Build history of the part. All positions in model axes, mm. Face numbers are marked on the shaded views. A direction names the side the tool comes from. Round coordinates to 2 decimals unless told otherwise and drop trailing zeros. Write each loop counter-clockwise with the first axis right and the second up, starting at its lowest first coordinate (ties: lowest second). Pieces come first, ordered by that corner, then holes. Notation, with made-up numbers: (-16.5, -31) - (-9.5, -31) arc R28 ccw to (-9.5, -6) - close; hole circle Ø3 at (60.5, 82). An arc over 180 degrees is marked (long way). One line per question, with ' | ' between items.
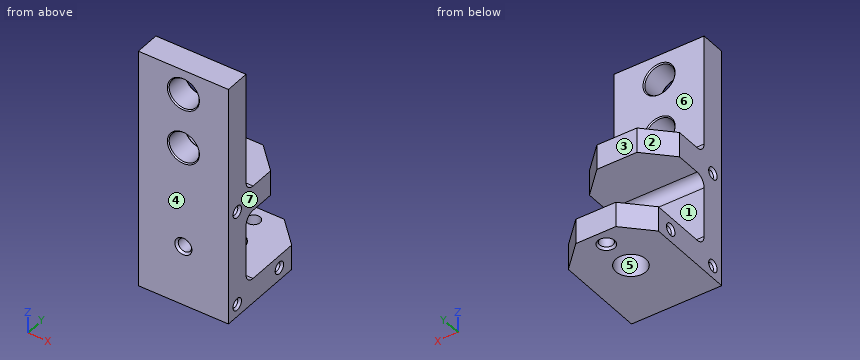
from build123d import *

# Parameters (mm, degrees)
EXTRUDE4_DEPTH                    = 57.15
EXTRUDE7_DEPTH                    = 57.15
CUT_EXTRUDE2_REACH                = 155.035
SKETCH10_R                        = 9.525
F_3_8_24_TAPPED_HOLE1_D           = 8.4328
F_3_8_24_TAPPED_HOLE1_DEPTH       = 15.875
F_3_8_24_TAPPED_HOLE1_CSINK_D     = 10.795
F_3_8_24_TAPPED_HOLE1_CSINK_ANGLE = 82
F_3_8_24_TAPPED_HOLE2_D           = 8.4328
F_3_8_24_TAPPED_HOLE2_DEPTH       = 15.875
F_3_8_24_TAPPED_HOLE2_CSINK_D     = 10.795
F_3_8_24_TAPPED_HOLE2_CSINK_ANGLE = 82
F_1_4_20_TAPPED_HOLE1_D           = 5.1054
F_1_4_20_TAPPED_HOLE1_DEPTH       = 16.51
F_1_4_20_TAPPED_HOLE1_CSINK_D     = 7.62
F_1_4_20_TAPPED_HOLE1_CSINK_ANGLE = 82
F_1_4_20_TAPPED_HOLE1_TIP         = 1.533816902
F_1_4_20_TAPPED_HOLE2_D           = 5.1054
F_1_4_20_TAPPED_HOLE2_DEPTH       = 16.51
F_1_4_20_TAPPED_HOLE2_CSINK_D     = 7.62
F_1_4_20_TAPPED_HOLE2_CSINK_ANGLE = 82
F_1_4_20_TAPPED_HOLE2_TIP         = 1.533816902
CUT_EXTRUDE3_REACH                = 155.035
F_1_2_CLEARANCE_HOLE1_AT_2_COUNT  = 2
F_1_2_CLEARANCE_HOLE1_AT_2_PITCH  = 34.925
CUT_EXTRUDE4_REACH                = 78.2
FILLET4_R                         = 6.35


with BuildPart() as part:
    # Sketch5 → Extrude4 (new body)
    with BuildSketch(Plane(origin=(0, 0, 0), x_dir=(0, 0, -1), z_dir=(1, 0, 0))):
        Polygon((0, 46.0375), (0, -7.9375), (-92.71, -7.9375), (-92.71, 7.9375), (-15.875, 7.9375), (-15.875, 46.0375), align=None)
    extrude(amount=EXTRUDE4_DEPTH)

    # Sketch9 → Extrude7 (add)
    with BuildSketch(Plane(origin=(57.15, 0, 0), x_dir=(0, 0, -1), z_dir=(1, 0, 0))):
        Polygon((0, 7.9375), (44.45, 7.9375), (44.45, 65.0875), (60.325, 65.0875), (60.325, -7.9375), (0, -7.9375), align=None)
    extrude(amount=-EXTRUDE7_DEPTH)

    # Sketch10 → Cut-Extrude2 (cut, up to next)
    with BuildSketch(Plane(origin=(0, 0, -60.325), x_dir=(-1, 0, 0), z_dir=(0, 0, -1)), mode=Mode.PRIVATE) as cut_extrude2_sk1:
        with Locations((-28.575, 33.3375)):
            Circle(SKETCH10_R)
    cut_extrude2_tool1 = extrude(cut_extrude2_sk1.sketch, amount=-CUT_EXTRUDE2_REACH, mode=Mode.PRIVATE) & part.part
    add(cut_extrude2_tool1.solids().sort_by_distance((28.575, 33.3375, -60.325))[0], mode=Mode.SUBTRACT)

    # 3/8-24 Tapped Hole1
    with Locations(Plane(origin=(0, 0, -60.325), x_dir=(-1, 0, 0), z_dir=(0, 0, -1))):
        with Locations((-28.575, 55.5625)):
            CounterSinkHole(F_3_8_24_TAPPED_HOLE1_D / 2, F_3_8_24_TAPPED_HOLE1_CSINK_D / 2, depth=F_3_8_24_TAPPED_HOLE1_DEPTH, counter_sink_angle=F_3_8_24_TAPPED_HOLE1_CSINK_ANGLE)

    # 3/8-24 Tapped Hole2
    with Locations(Plane.XZ.offset(7.9375)):
        with Locations((28.575, -22.225)):
            CounterSinkHole(F_3_8_24_TAPPED_HOLE2_D / 2, F_3_8_24_TAPPED_HOLE2_CSINK_D / 2, depth=F_3_8_24_TAPPED_HOLE2_DEPTH, counter_sink_angle=F_3_8_24_TAPPED_HOLE2_CSINK_ANGLE)

    # 1/4-20 Tapped Hole1
    with Locations(Plane.ZY):
        with Locations((-52.3875, 0), (7.9375, 0), (-52.3875, 38.1)):
            CounterSinkHole(F_1_4_20_TAPPED_HOLE1_D / 2, F_1_4_20_TAPPED_HOLE1_CSINK_D / 2, depth=F_1_4_20_TAPPED_HOLE1_DEPTH, counter_sink_angle=F_1_4_20_TAPPED_HOLE1_CSINK_ANGLE)
            with Locations((0, 0, -(F_1_4_20_TAPPED_HOLE1_DEPTH + F_1_4_20_TAPPED_HOLE1_TIP / 2))):  # 118° drill point
                Cone(0, F_1_4_20_TAPPED_HOLE1_D / 2, F_1_4_20_TAPPED_HOLE1_TIP, mode=Mode.SUBTRACT)

    # 1/4-20 Tapped Hole2
    with Locations(Plane(origin=(57.15, 0, 0), x_dir=(0, 0, -1), z_dir=(1, 0, 0))):
        with Locations((52.3875, 0), (-7.9375, 0), (52.3875, 38.1)):
            CounterSinkHole(F_1_4_20_TAPPED_HOLE2_D / 2, F_1_4_20_TAPPED_HOLE2_CSINK_D / 2, depth=F_1_4_20_TAPPED_HOLE2_DEPTH, counter_sink_angle=F_1_4_20_TAPPED_HOLE2_CSINK_ANGLE)
            with Locations((0, 0, -(F_1_4_20_TAPPED_HOLE2_DEPTH + F_1_4_20_TAPPED_HOLE2_TIP / 2))):  # 118° drill point
                Cone(0, F_1_4_20_TAPPED_HOLE2_D / 2, F_1_4_20_TAPPED_HOLE2_TIP, mode=Mode.SUBTRACT)

    # Sketch19 → Cut-Extrude3 (cut, up to next)
    with BuildSketch(Plane(origin=(0, 0, -60.325), x_dir=(-1, 0, 0), z_dir=(0, 0, -1)), mode=Mode.PRIVATE) as cut_extrude3_sk1:
        Polygon((-57.15, 49.2125), (-41.275, 65.0875), (-57.15, 65.0875), align=None)
    cut_extrude3_tool1 = extrude(cut_extrude3_sk1.sketch, amount=-CUT_EXTRUDE3_REACH, mode=Mode.PRIVATE) & part.part
    add(cut_extrude3_tool1.solids().sort_by_distance((51.858333, 59.795833, -60.325))[0], mode=Mode.SUBTRACT)
    # Sketch19 → Cut-Extrude3 (cut, up to next)
    with BuildSketch(Plane(origin=(0, 0, -60.325), x_dir=(-1, 0, 0), z_dir=(0, 0, -1)), mode=Mode.PRIVATE) as cut_extrude3_sk2:
        Polygon((0, 49.2125), (0, 65.0875), (-15.875, 65.0875), align=None)
    cut_extrude3_tool2 = extrude(cut_extrude3_sk2.sketch, amount=-CUT_EXTRUDE3_REACH, mode=Mode.PRIVATE) & part.part
    add(cut_extrude3_tool2.solids().sort_by_distance((5.291667, 59.795833, -60.325))[0], mode=Mode.SUBTRACT)

    # Sketch22 → 1/2 Clearance Hole1 (revolve, cut)
    with BuildSketch(Plane(origin=(28.575, -7.9375, 77.0255), x_dir=(0, 0, -1), z_dir=(1, 0, 0))):
        Polygon((0, 0), (0, 15.875), (10.16, 15.875), (9.525, 15.144516061), (9.525, 0.730483939), (10.16, 0), align=None)
    f_1_2_clearance_hole1 = revolve(axis=Axis((28.575, -14.2875, 77.0255), (0, 1, 0)), mode=Mode.SUBTRACT)

    # 1/2 Clearance Hole1 at 2: 1/2 Clearance Hole1 ×2
    with Locations(*[(0, 0, -i * F_1_2_CLEARANCE_HOLE1_AT_2_PITCH) for i in range(1, F_1_2_CLEARANCE_HOLE1_AT_2_COUNT)]):
        add(f_1_2_clearance_hole1, mode=Mode.SUBTRACT)

    # Sketch24 → Cut-Extrude4 (cut, up to next)
    with BuildSketch(Plane.XY.offset(15.875), mode=Mode.PRIVATE) as cut_extrude4_sk1:
        Polygon((0, 30.1625), (15.875, 46.0375), (0, 46.0375), align=None)
    cut_extrude4_tool1 = extrude(cut_extrude4_sk1.sketch, amount=-CUT_EXTRUDE4_REACH, mode=Mode.PRIVATE) & part.part
    add(cut_extrude4_tool1.solids().sort_by_distance((5.291667, 40.745833, 15.875))[0], mode=Mode.SUBTRACT)
    # Sketch24 → Cut-Extrude4 (cut, up to next)
    with BuildSketch(Plane.XY.offset(15.875), mode=Mode.PRIVATE) as cut_extrude4_sk2:
        Polygon((57.15, 30.1625), (57.15, 46.0375), (41.275, 46.0375), align=None)
    cut_extrude4_tool2 = extrude(cut_extrude4_sk2.sketch, amount=-CUT_EXTRUDE4_REACH, mode=Mode.PRIVATE) & part.part
    add(cut_extrude4_tool2.solids().sort_by_distance((51.858333, 40.745833, 15.875))[0], mode=Mode.SUBTRACT)

    # Fillet4
    fillet4_edges = [part.edges().sort_by_distance(p)[0] for p in [
        (28.575, 7.9375, 0),
        (28.575, 7.9375, -44.45),
        (28.575, 7.9375, 15.875),
    ]]
    fillet(fillet4_edges, radius=FILLET4_R)


solid = part.part
Q1. Which spindle directions (+Z, -Z, +X, -X, +Y, -Y) get a long thin tool onto all of the face, cutting with end or side? Do the marked faces 1, 2, 3 and 4. Say none if no direction does.
Found:
face 1: +X, -X, +Y | face 2: +Z, -X, +Y | face 3: +Z, +X, -X, +Y | face 4: +Z, -Z, +X, -X, -Y
Q2. Drop flat-ended pins along their axis: pin 1 (4.5 mm diameter, centred on y = 0, z = -52.39, fed in from +X); pin 2 (1.5 mm diameter, centred on x = 26.5, z = -2.5, fed in from +Y); pin 3 (4 mm diameter, centred on y = 38.1, z = -52.39, fed in from +X); pin 4 (6.5 mm diameter, centred on x = 28.575, z = -22.225, fed in from +Y). Give the stop position or say it passes through.
Found:
pin 1: x = 40.46 | pin 2: y = 9.91 | pin 3: x = 40.31 | pin 4: through
Q3. Pull direction X, two halves, no side cores. Call the marked faces 5, 6 and 7: +X half, -X half, draft (parallel to the pull), parting line (faces both ways), or undercut.
Found:
face 5: undercut | face 6: draft | face 7: +X half
Q4. Drill centre lines: L1, parallel to Z at x = 11, y = 0 (3 decimals); L2, parallel to Z at x = 37.5, y = 15 (3 decimals); L3, parallel to Z at x = 20.5, y = 37.5 (3 decimals). Where is each one in solid material? Low to high. Write a range as from..to.
Found:
L1: -60.325..-54.94, -49.835..5.385, 10.49..92.71 | L2: -60.325..-44.45, 0..15.875 | L3: 0..15.875
Q5. Saw through at B-B, the plane z = -11. List the corners of the cut face in (x, y), then the cut area to 3 significant figures.
Found:
outline: (0, -7.94) - (57.15, -7.94) - (57.15, 7.94) - (0, 7.94) - close | area: 907 mm^2
Q6. Saw through at A-A, the plane x = 7. State how many separate pieces and enclosed holes the cut face has, then the cut area to 3 significant figures.
Found:
separate pieces: 1 | enclosed holes: 3 | area: 3,620 mm^2
